```python
from build123d import *

# Parameters (mm, degrees)
BOSS_EXTRUDE1_DEPTH = 6.35
FILLET1_R           = 10
SKETCH2_R           = 2.8702
CUT_EXTRUDE1_DEPTH  = 81.739915371


with BuildPart() as part:
    # Sketch1 → Boss-Extrude1 (new body)
    with BuildSketch(Plane.XY):
        Polygon((26.235565231, 15.475), (38.935565231, 15.475), (38.935565231, 9.125), (51.635565231, 9.125), (51.635565231, 15.475), (64.335565231, 15.475), (64.335565231, 9.125), (78.988200442, 9.125), (78.988200442, -9.925), (-35.311799558, -9.925), (-35.311799558, 9.125), (26.235565231, 9.125), align=None)
    extrude(amount=BOSS_EXTRUDE1_DEPTH)

    # Fillet1
    # the kernel refuses this fillet: 10 mm, written as the material it takes off along each edge
    with BuildSketch(Plane(origin=(78.988200442, -9.925, -25), x_dir=(0, 1, 0), z_dir=(0, 0, 1)), Plane(origin=(-35.311799558, 9.125, -25), x_dir=(0, -1, 0), z_dir=(0, 0, 1)), Plane(origin=(-35.311799558, -9.925, -25), x_dir=(1, 0, 0), z_dir=(0, 0, 1))) as fillet1_piece_1:
        with BuildLine():
            CenterArc((FILLET1_R, FILLET1_R), FILLET1_R, 180, 90)
            Line((0, FILLET1_R), (0, 0))
            Line((0, 0), (FILLET1_R, 0))
        make_face()
    extrude(amount=56.35, mode=Mode.SUBTRACT)

    # Sketch2 → Cut-Extrude1 (cut, through all)
    with BuildSketch(Plane.XY.offset(6.35)):
        Circle(SKETCH2_R)
    extrude(amount=-CUT_EXTRUDE1_DEPTH, mode=Mode.SUBTRACT)


solid = part.part
```
Geometry check sheet. Reference: the model listing, model coordinates, mm. A direction names the side the tool comes from. Round coordinates to 2 decimals unless told otherwise and drop trailing zeros. Loops run counter-clockwise (first coordinate to the right, second up) from the corner with the lowest first, then second, coordinate; pieces in that order, holes last. Notation, with made-up numbers: (17, -2.5) - (40, -2.5) arc R22 ccw to (40, 20.5) - close; hole circle Ø1 at (-1.75, 63.5). An arc over 180 degrees is marked (long way). Write each question's results on one line, items separated by ' | '. Start each with the question number.
Q1. Release check for a two-part mould opening along Y. For faces 6 (the cylindrical face through (-2.278, -1.746, 3.219)), 7 (the flat face through (72, 9.125, 3)), 8 (the flat face through (26.236, 12, 3)) record: +Y half, -Y half, draft (parallel to the pull), parting line (faces both ways), or undercut.
Q2. Gauge pin test, flat ends, axial feed: P1, Ø1.9, axis at x = 44, z = 4.5, coming from the +Y side (3 decimals); P2, Ø1.5, axis at y = 3, z = 5, coming from the -X side; P3, Ø1.9, axis at y = 12.5, z = 2.5, coming from the +X side. Record the tip position at first contact, or that the pin passes through.
Q3. Cross-section at B-B on z = 1.75. Enter the section's corners in (x, y) (3 decimals).
Q4. Thickness scan on line 1 (Y direction, x = 0, z = 2) (3 decimals); line 2 (X direction, y = 11.25, z = 3.5); line 3 (Y direction, x = 68, z = 5) (3 decimals). Record the ranges inside material, lowest first. Write a range as [from, to].
Q5. Cross-section at D-D on x = -12.5. Enter the section's corners in (y, z) (3 decimals).
Q6. Access from +Z, -Z, +X, -X, +Y, -Y to the whole of each face (thin tool, end or side, straight path). Record for faces 1 (the flat face through (32, 15.475, 3)), 2 (the flat face through (45, 9.125, 3)), 3 (the flat face through (0, 9.125, 3)), 4 (the flat face through (64.336, 12, 3)), 5 (the flat face through (23, 0, 0)).
Q7. Cross-section at A-A on x = 0. Enter the section's corners in (y, z) (3 decimals).
Q8. Cross-section at C-C on y = 1.5. Enter the section's corners in (x, z), and give its area (3 significant figures).
Answers below:
1) face 6: undercut | face 7: +Y half | face 8: draft
2) P1: stops at y = 9.125 | P2: stops at x = -34.81 | P3: stops at x = 64.34
3) outline: (-35.301, -0.4) arc R10 ccw to (-25.312, -9.925) - (68.988, -9.925) arc R10 ccw to (78.988, 0.075) - (78.988, 9.125) - (64.336, 9.125) - (64.336, 15.475) - (51.636, 15.475) - (51.636, 9.125) - (38.936, 9.125) - (38.936, 15.475) - (26.236, 15.475) - (26.236, 9.125) - (-25.312, 9.125) arc R10 ccw to start; hole circle Ø5.74 at (0, 0)
4) line 1: y = [-9.925, -2.87], [2.87, 9.125] | line 2: x = [26.24, 38.94], [51.64, 64.34] | line 3: y = [-9.925, 9.125]
5) outline: (-9.925, 0) - (9.125, 0) - (9.125, 6.35) - (-9.925, 6.35) - close
6) face 1: +Z, -Z, +X, -X, +Y | face 2: +Z, -Z, +Y | face 3: +Z, -Z, -X, +Y | face 4: +Z, -Z, +X, +Y | face 5: -Z, +X, -X, +Y, -Y
7) outline: (-9.925, 0) - (-2.87, 0) - (-2.87, 6.35) - (-9.925, 6.35) - close; (2.87, 0) - (9.125, 0) - (9.125, 6.35) - (2.87, 6.35) - close
8) outline: (-35.03, 0) - (-2.45, 0) - (-2.45, 6.35) - (-35.03, 6.35) - close; (2.45, 0) - (78.99, 0) - (78.99, 6.35) - (2.45, 6.35) - close | area: 693 mm²
